Geometry check sheet. Reference: the model listing, model coordinates, mm. Face numbers are marked on the shaded views. A direction names the side the tool comes from. Coordinates: 2 decimals unless noted, no trailing zeros. Write each loop counter-clockwise with the first axis right and the second up, starting at its lowest first coordinate (ties: lowest second). Pieces come first, ordered by that corner, then holes.
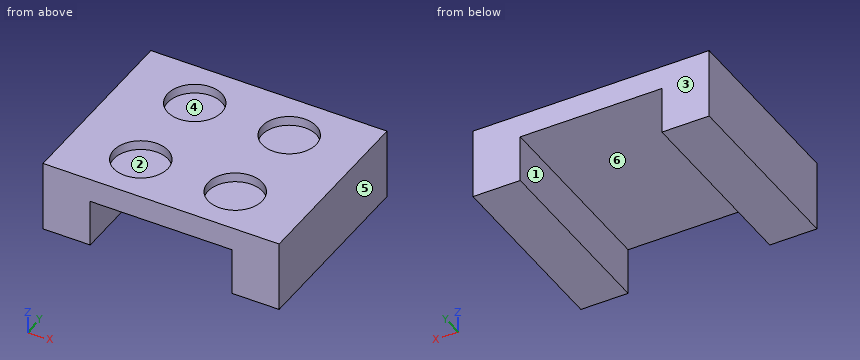
from build123d import *

# Parameters (mm, degrees)
EXTRUDE_1_DEPTH     = 40
SKETCH_2_R          = 5.75
CUT_EXTRUDE_1_DEPTH = 2


with BuildPart() as part:
    # 草图1 → 凸台-拉伸1 (new body)
    with BuildSketch(Plane(origin=(0, 0, 0), x_dir=(1, 0, 0), z_dir=(0, 1, 0))):
        Polygon((0, 0), (0, -15), (50, -15), (50, 0), (40, 0), (40, -10), (10, -10), (10, 0), align=None)
    extrude(amount=EXTRUDE_1_DEPTH)

    # 草图2 → 切除-拉伸1 (cut)
    with BuildSketch(Plane.XY.offset(15)):
        with Locations((15, 30)):
            Circle(SKETCH_2_R)
        with Locations((35, 30)):
            Circle(SKETCH_2_R)
        with Locations((15, 10)):
            Circle(SKETCH_2_R)
        with Locations((35, 10)):
            Circle(SKETCH_2_R)
    extrude(amount=-CUT_EXTRUDE_1_DEPTH, mode=Mode.SUBTRACT)


solid = part.part
1. Sectioned sample at C-C, the plane x = 15. Record the boundary of the cut face in (y, z).
Computed values:
outline: (0, 10) - (40, 10) - (40, 15) - (35.75, 15) - (35.75, 13) - (24.25, 13) - (24.25, 15) - (15.75, 15) - (15.75, 13) - (4.25, 13) - (4.25, 15) - (0, 15) - close
2. Gauge pin test, flat ends, axial feed: pin 1 Ø10.5 at (x, y) = (15, 10) entering from +Z; pin 2 Ø6 at (x, y) = (20.5, 22.5) entering from -Z. Record the tip position at first contact, or that the pin passes through.
Computed values:
pin 1: stops at z = 13
pin 2: stops at z = 10
3. Sectioned sample at B-B, the plane y = 38.5. Record the boundary of the cut face in (x, z).
Computed values:
outline: (0, 0) - (10, 0) - (10, 10) - (40, 10) - (40, 0) - (50, 0) - (50, 15) - (0, 15) - close
4. Draft check along Y on the marked faces 1, 2 and 3. Enter one of: released by +Y, released by -Y, zero draft, split by the parting line, or undercut.
Computed values:
face 1: zero draft
face 2: undercut
face 3: released by +Y
5. Thickness scan on line 1 along Y through (x, z) = (15, 13.4); line 2 along X through (y, z) = (10.5, 9.75); line 3 along Z through (x, y) = (21, 6). Record the ranges inside material, lowest first.
Computed values:
line 1: y = 0 to 4.25, 15.75 to 24.25, 35.75 to 40
line 2: x = 0 to 10, 40 to 50
line 3: z = 10 to 15
6. Sectioned sample at A-A, the plane z = 5. Record the boundary of the cut face in (x, y), and give its area (3 significant figures).
Computed values:
outline: (0, 0) - (10, 0) - (10, 40) - (0, 40) - close; (40, 0) - (50, 0) - (50, 40) - (40, 40) - close
area: 800 mm2
7. Sectioned sample at D-D, the plane y = 30. Record the boundary of the cut face in (x, z), and give its area (3 significant figures).
Computed values:
outline: (0, 0) - (10, 0) - (10, 10) - (40, 10) - (40, 0) - (50, 0) - (50, 15) - (40.75, 15) - (40.75, 13) - (29.25, 13) - (29.25, 15) - (20.75, 15) - (20.75, 13) - (9.25, 13) - (9.25, 15) - (0, 15) - close
area: 404 mm2
8. Access from +Z, -Z, +X, -X, +Y, -Y to the whole of each face (thin tool, end or side, straight path). Record for the marked faces 4, 5 and 6.
Computed values:
face 4: +Z
face 5: +Z, -Z, +X, +Y, -Y
face 6: -Z, +Y, -Y
